```python
from build123d import *

# Parameters (mm, degrees)
F1_DEPTH = 1
F2_R     = 1
F3_DEPTH = 2
F4_W     = 28
F4_H     = 28
F4_W_2   = 14.5
F4_H_2   = 14.5
F5_DEPTH = 2.5
F6_R     = 0.5
F7_W     = 9.5
F7_H     = 13.5
F8_DEPTH = 1


with BuildPart() as f1:
    # F0 (on Top) → F1 (new body)
    with BuildSketch(Plane.XY):
        Polygon((-41.764005, 41.031135), (-41.764005, -58.968865), (-11.764005, -58.968865), (34.235995, 4.031135), (34.235995, 41.031135), align=None)
    extrude(amount=F1_DEPTH)

    # F2 (on face) → F3 (cut)
    with BuildSketch(Plane.XY.offset(1)):
        with Locations((-28.664005, 26.031135)):
            Circle(F2_R)
        with Locations((-28.664005, -15.868865)):
            Circle(F2_R)
        with Locations((29.035995, 26.031135)):
            Circle(F2_R)
        with Locations((-1.764005, -40.168865)):
            Circle(F2_R)
    extrude(amount=-F3_DEPTH, mode=Mode.SUBTRACT)

    # F4 (on face) → F5 (join)
    with BuildSketch(Plane.XY.offset(1)):
        with Locations((-11.764005, 2.031135)):
            Rectangle(F4_W, F4_H)
        with Locations((12.985995, 4.281135)):
            Rectangle(F4_W_2, F4_H_2)
    extrude(amount=F5_DEPTH)

    # F6
    f6_edges = [f1.edges().sort_by_distance(p)[0] for p in [
        (-11.764005, -11.968865, 3.5),
        (-25.764005, 2.031135, 3.5),
        (-11.764005, 16.031135, 3.5),
        (2.235995, 2.031135, 3.5),
        (12.985995, 11.531135, 3.5),
        (5.735995, 4.281135, 3.5),
        (12.985995, -2.968865, 3.5),
        (20.235995, 4.281135, 3.5),
    ]]
    fillet(f6_edges, radius=F6_R)

    # F7 (on face) → F8 (join)
    with BuildSketch(Plane.XY.offset(1)):
        with Locations((-15.014005, -23.218865)):
            Rectangle(F7_W, F7_H)
    extrude(amount=F8_DEPTH)


solid = f1.part
```
Geometry: final body of the model. Coordinates: model frame, mm. A direction names the side the tool comes from. Coordinates: 2 decimals unless noted, no trailing zeros. Order: outer loops, then holes, each group sorted by start corner. A loop starts at its lowest first (then second) coordinate and runs counter-clockwise, first axis right, second up.
Item 1: Section query A-A (y = 7.5). Output: boundary loops of the cut face in (x, z).
Answer:
outline: (-41.76, 0) - (34.24, 0) - (34.24, 1) - (20.24, 1) - (20.24, 3) arc R0.5 ccw to (19.74, 3.5) - (6.24, 3.5) arc R0.5 ccw to (5.74, 3) - (5.74, 1) - (2.24, 1) - (2.24, 3) arc R0.5 ccw to (1.74, 3.5) - (-25.26, 3.5) arc R0.5 ccw to (-25.76, 3) - (-25.76, 1) - (-41.76, 1) - close
Item 2: Draft query along Y for faces 1 (the face through (10.914, -27.91, 0.493)), 2 (the face through (-1.894, -39.177, 0.507)), 3 (the face through (2.236, 2, 2)), 4 (the face through (13, 11.531, 2)). Return one class per face: released by +Y, released by -Y, zero draft, split by the parting line, or undercut.
Answer:
face 1: released by -Y
face 2: undercut
face 3: zero draft
face 4: released by +Y
Item 3: Contact query for flat-ended pins moving along their axis: P1, Ø1, axis at x = 19, y = 13, coming from the +Z side; P2, Ø0.8, axis at y = -21, z = 1.5, coming from the +X side; P3, Ø8, axis at x = 18, y = -11.5, coming from the -Z side; P4, Ø0.8, axis at x = -15.5, z = 1.5, coming from the +Y side. Output: stop coordinate, or through.
Answer:
P1: stops at z = 1
P2: stops at x = -10.26
P3: stops at z = 0
P4: stops at y = 16.03
Item 4: Material intervals for line 1 along X through (y, z) = (-4.5, 2.65); line 2 along Z through (x, y) = (-13, -48); line 3 along X through (y, z) = (-27.5, 1.85), sorted ascending.
Answer:
line 1: x = -25.76 to 2.24
line 2: z = 0 to 1
line 3: x = -19.76 to -10.26
Item 5: Section query D-D (x = 0.5). Output: boundary loops of the cut face in (y, z).
Answer:
outline: (-42.17, 0) - (41.03, 0) - (41.03, 1) - (16.03, 1) - (16.03, 3) arc R0.5 ccw to (15.53, 3.5) - (-11.47, 3.5) arc R0.5 ccw to (-11.97, 3) - (-11.97, 1) - (-42.17, 1) - close
Item 6: Section query B-B (x = -17). Output: boundary loops of the cut face in (y, z).
Answer:
outline: (-58.97, 0) - (41.03, 0) - (41.03, 1) - (16.03, 1) - (16.03, 3) arc R0.5 ccw to (15.53, 3.5) - (-11.47, 3.5) arc R0.5 ccw to (-11.97, 3) - (-11.97, 1) - (-16.47, 1) - (-16.47, 2) - (-29.97, 2) - (-29.97, 1) - (-58.97, 1) - close
Item 7: Section query C-C (y = -5). Output: boundary loops of the cut face in (x, z), then the cut area to 3 significant figures.
Answer:
outline: (-41.76, 0) - (27.64, 0) - (27.64, 1) - (2.24, 1) - (2.24, 3) arc R0.5 ccw to (1.74, 3.5) - (-25.26, 3.5) arc R0.5 ccw to (-25.76, 3) - (-25.76, 1) - (-41.76, 1) - close
area: 139 mm2
Item 8: Access query for faces 5 (the face through (-25.764, 2, 2)), 6 (the face through (-15, -23, 2)), 7 (the face through (-12, 16.031, 2)), 8 (the face through (13, -2.969, 2)), 9 (the face through (20.236, 4, 2)). Directions: +Z, -Z, +X, -X, +Y, -Y. A direction counts if a zero-diameter tool reaches every point of the face in a straight line with its end or side. Return the directions, or none.
Answer:
face 5: +Z, -X, +Y, -Y
face 6: +Z, +X, -X, -Y
face 7: +Z, +X, -X, +Y
face 8: +Z, +X, -Y
face 9: +Z, +X, +Y, -Y
